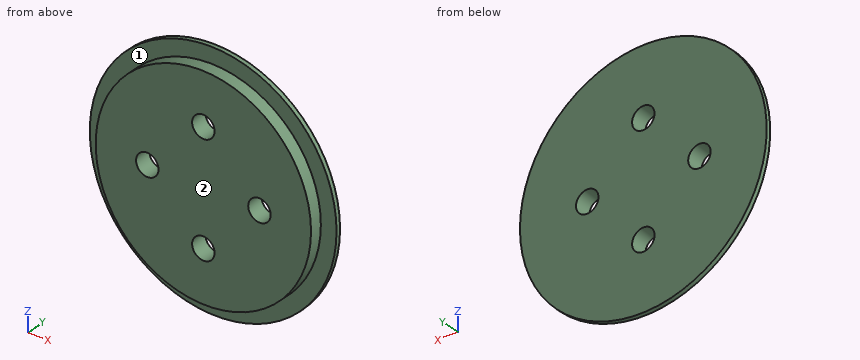
```python
from build123d import *

# Parameters (mm, degrees)
F0_R     = 55
F1_DEPTH = 2
F2_R     = 48
F3_DEPTH = 5.6
F5_D     = 10


with BuildPart() as f1:
    # F0 (on Front) → F1 (new body)
    with BuildSketch(Plane.XZ):
        Circle(F0_R)
    extrude(amount=F1_DEPTH)

    # F2 (on face) → F3 (join)
    with BuildSketch(Plane.XZ.offset(2)):
        Circle(F2_R)
    extrude(amount=F3_DEPTH)

    # F5 (through all)
    with Locations(Plane.XZ.offset(7.6)):
        with Locations((-25, 0), (0, 25), (25, 0), (0, -25)):
            Hole(F5_D / 2)


solid = f1.part
```
Geometry: final body of the model. Coordinates: model frame, mm. Face numbers are marked on the shaded views. A direction names the side the tool comes from. Coordinates: 2 decimals unless noted, no trailing zeros. Loops run counter-clockwise (first coordinate to the right, second up) from the corner with the lowest first, then second, coordinate; pieces in that order, holes last. Notation, with made-up numbers: (32.25, 14) -> (61.25, 14) arc R22 ccw to (61.25, 50) -> close; hole circle Ø11 at (36.25, 46.5). An arc over 180 degrees is marked (long way). Use a Markdown table: item, result. Add a question column.
(1) Access query for the marked faces 1 and 2. Directions: +Z, -Z, +X, -X, +Y, -Y. A direction counts if a zero-diameter tool reaches every point of the face in a straight line with its end or side. Return the directions, or none.
(2) Pin query (flat end, axial travel): pin 1 Ø11.5 at (x, z) = (25, 0) entering from +Y; pin 2 Ø2 at (y, z) = (-6.5, 30) entering from +X. Return the tip coordinate at first contact, or that it passes through.
(3) Section query B-B, the plane x = 2. Return loops of the section in (y, z).
(4) Section query D-D, the plane y = -5.5. Return loops of the section in (x, z), plus the area to 3 significant figures.
(5) Line query: line 1 along Z through (x, y) = (0, -5.5); line 2 along X through (y, z) = (-3.5, -3.5); line 3 along Z through (x, y) = (-4.5, -2.5). Output: solid intervals per line, ascending.
(6) Section query C-C, the plane x = -28. Return loops of the section in (y, z).
(7) Section query A-A, the plane z = 0. Return loops of the section in (x, y), plus the area to 3 significant figures.
Answer:
| question | item | result |
|---|---|---|
| 1 | face 1 | -Y |
| 1 | face 2 | +Z, -Z, +X, -X, -Y |
| 2 | pin 1 | stops at y = 0 |
| 2 | pin 2 | stops at x = 38.25 |
| 3 | outline | (-7.6, -47.96) -> (-2, -47.96) -> (-2, -54.96) -> (0, -54.96) -> (0, -29.58) -> (-7.6, -29.58) -> close; (-7.6, -20.42) -> (0, -20.42) -> (0, 20.42) -> (-7.6, 20.42) -> close; (-7.6, 29.58) -> (0, 29.58) -> (0, 54.96) -> (-2, 54.96) -> (-2, 47.96) -> (-7.6, 47.96) -> close |
| 4 | outline | circle Ø96 at (0, 0); hole circle Ø10 at (-25, 0); hole circle Ø10 at (0, -25); hole circle Ø10 at (0, 25); hole circle Ø10 at (25, 0) |
| 4 | area | 6,920 mm^2 |
| 5 | line 1 | z = -48 to -30, -20 to 20, 30 to 48 |
| 5 | line 2 | x = -47.87 to -28.57, -21.43 to 21.43, 28.57 to 47.87 |
| 5 | line 3 | z = -47.79 to -27.18, -22.82 to 22.82, 27.18 to 47.79 |
| 6 | outline | (-7.6, -38.99) -> (-2, -38.99) -> (-2, -47.34) -> (0, -47.34) -> (0, -4) -> (-7.6, -4) -> close; (-7.6, 4) -> (0, 4) -> (0, 47.34) -> (-2, 47.34) -> (-2, 38.99) -> (-7.6, 38.99) -> close |
| 7 | outline | (-55, -2) -> (-48, -2) -> (-48, -7.6) -> (-30, -7.6) -> (-30, 0) -> (-55, 0) -> close; (-20, -7.6) -> (20, -7.6) -> (20, 0) -> (-20, 0) -> close; (30, -7.6) -> (48, -7.6) -> (48, -2) -> (55, -2) -> (55, 0) -> (30, 0) -> close |
| 7 | area | 606 mm^2 |
